Build history of the part. All positions in model axes, mm. A direction names the side the tool comes from. Give positions to 0.01 mm unless a question says otherwise; leave off trailing zeros. Write each loop counter-clockwise with the first axis right and the second up, starting at its lowest first coordinate (ties: lowest second). Pieces come first, ordered by that corner, then holes. Notation, with made-up numbers: M 15.25,7.25 L 36.25,7.25 A17 ccw 36.25,20.25 Z; hole C 0,-20.5 d4. An arc over 180 degrees is marked long. Return JSON: item names as keys, results as strings. Group by question number.
Q1. Band-saw the part on C-C, the plane y = 9.5. Give the cut face in (x, z), then the cut area to 3 significant figures.
Q2. Band-saw the part on A-A, the plane z = 0. Give the cut face in (x, y).
Q3. Tool access for faces 4 (the flat face through (-15, 6, -7.85)), 5 (the flat face through (-30, -8, 0)), 6 (the flat face through (-38.898, -8.874, 40.373)), 7 (the flat face through (-25, -15.35, 43)), 8 (the flat face through (-28.577, 15, -3)): list every direction of +Z, -Z, +X, -X, +Y, -Y with a clear straight run to the whole face (end or side of a thin tool).
Q4. Band-saw the part on B-B, the plane y = 20. Give the cut face in (x, z), then the cut area to 3 significant figures.
Q5. Band-saw the part on D-D, the plane z = 17.5. Give the cut face in (x, y), then the cut area to 3 significant figures.
Q6. Flat gauge pins, fed straight in: pin 1 Ø2 at (x, z) = (-16.5, 29) entering from +Y; pin 2 Ø7.5 at (x, y) = (-47.5, -6.5) entering from +Z; pin 3 Ø4 at (x, y) = (-40, -7.5) entering from +Z; pin 4 Ø4 at (y, z) = (2.5, 58) entering from -X. Where does each tip first touch, or does it go through?
Q7. Wall check: probe 1 along Z at (x, y) = (-4.95, 20); probe 2 along Z at (x, y) = (-44.5, -10); probe 3 along Y at (x, z) = (-60, -8.85). Give the ranges that are in metal, low to high.
Q8. Pull direction X, two halves, no side cores. Call faces 1 (the cylindrical face through (-5.43, -6.5, 0.07)), 2 (the flat face through (-42.943, -2.465, 53.109)), 3 (the cylindrical face through (-12.39, -7.3, 40.75)): +X half, -X half, draft (parallel to the pull), parting line (faces both ways), or undercut.
from build123d import *

# Parameters (mm, degrees)
F0_W      = 15
F0_H      = 15
F1_DEPTH  = 15
F2_W      = 15
F2_H      = 15
F3_DEPTH  = 3
F5_DEPTH  = 30
F6_R      = 1.5
F7_DEPTH  = 6.001
F8_R      = 1.5
F9_DEPTH  = 24.8215080757
F10_R     = 1.5
F11_DEPTH = 6.001
F12_SIZE  = 5
F13_SIZE  = 2
F14_W     = 15.7
F14_H     = 15.7
F15_DEPTH = 48.001
F16_W     = 15.7
F16_H     = 15.7
F17_DEPTH = 63.3466714755
F18_W     = 15.7
F18_H     = 15.7
F19_DEPTH = 40.001
F21_DEPTH = 18.001


with BuildPart() as f1:
    # F0 (on Front) → F1 (new body)
    with BuildSketch(Plane.XZ):
        Polygon((-70, 7.5), (-30, 7.5), (-30, -7.5), (-70, -7.5), (-70, -13.5), (-1.5766062413, -13.5), (-1.5766062413, 29.7307621135), (-23.3086570489, 67.3717782649), (-28.5048094716, 64.3717782649), (-8.5048094716, 29.7307621135), (-21.4951905284, 22.2307621135), (-41.4951905284, 56.8717782649), (-46.6913429511, 53.8717782649), (-30.8826859022, 26.4903810568), (-38.3826859022, 13.5), (-70, 13.5), align=None)
        with Locations((-15.0766062413, 0)):
            Rectangle(F0_W, F0_H, mode=Mode.SUBTRACT)
    extrude(amount=F1_DEPTH)

    # F2 (on face) → F3 (join)
    with BuildSketch(Plane.XZ.offset(15)):
        Polygon((-38.3826859022, 13.5), (-70, 13.5), (-70, -13.5), (-1.5766062413, -13.5), (-1.5766062413, 29.7307621135), (-23.3086570489, 67.3717782649), (-46.6913429511, 53.8717782649), (-30.8826859022, 26.4903810568), align=None)
        with Locations((-15.0766062413, 0)):
            Rectangle(F2_W, F2_H, mode=Mode.SUBTRACT)
    extrude(amount=F3_DEPTH)

    # F4 (on face) → F5 (join)
    with BuildSketch(Plane(origin=(0, 0, 0), x_dir=(-1, 0, 0), z_dir=(0, 1, 0))):
        Polygon((7.5766062413, -7.5), (7.5766062413, 7.5), (1.5766062413, 7.5), (1.5766062413, -13.5), (28.5766062413, -13.5), (28.5766062413, 7.5), (22.5766062413, 7.5), (22.5766062413, -7.5), align=None)
    extrude(amount=F5_DEPTH)

    # F6 (on face) → F7 (cut, through all)
    with BuildSketch(Plane.XY.offset(-7.5)):
        with Locations((-40, -7.5)):
            Circle(F6_R)
        with Locations((-60, -7.5)):
            Circle(F6_R)
    extrude(amount=-F7_DEPTH, mode=Mode.SUBTRACT)

    # F8 (on face) → F9 (cut, through all)
    with BuildSketch(Plane(origin=(6.4951905284, 0, 3.75), x_dir=(0, -1, 0), z_dir=(-0.8660254038, 0, -0.5))):
        with Locations((7.5, 40)):
            Circle(F8_R)
        with Locations((7.5, 60)):
            Circle(F8_R)
    extrude(amount=-F9_DEPTH, mode=Mode.SUBTRACT)

    # F10 (on face) → F11 (cut, through all)
    with BuildSketch(Plane(origin=(-7.5766062413, 0, 0), x_dir=(0, -1, 0), z_dir=(-1, 0, 0))):
        with Locations((-20, 0)):
            Circle(F10_R)
        with Locations((8, 0)):
            Circle(F10_R)
    extrude(amount=-F11_DEPTH, mode=Mode.SUBTRACT)

    # F12
    f12_edges = [f1.edges().sort_by_distance(p)[0] for p in [
        (-25.906733, 0, 65.871778),
        (-44.093267, 0, 55.371778),
        (-4.576606, 30, 7.5),
        (-25.576606, 30, 7.5),
        (-70, 0, 10.5),
        (-70, 0, -10.5),
    ]]
    chamfer(f12_edges, length=F12_SIZE)

    # F13
    f13_edges = [f1.edges().sort_by_distance(p)[0] for p in [
        (-1.576606, -6.5, 0),
        (-1.576606, 21.5, 0),
        (-8.308657, -6, 41.391016),
        (-18.308657, -6, 58.711524),
        (-41.5, -7.5, -13.5),
        (-61.5, -7.5, -13.5),
    ]]
    chamfer(f13_edges, length=F13_SIZE)

    # F14 (on face) → F15 (cut, through all)
    with BuildSketch(Plane.XZ.offset(18)):
        with Locations((-15.0766062413, 0)):
            Rectangle(F14_W, F14_H)
    extrude(amount=-F15_DEPTH, mode=Mode.SUBTRACT)

    # F16 (on face) → F17 (cut, through all)
    with BuildSketch(Plane(origin=(-15, 0, 25.9807621135), x_dir=(0.8660254038, 0, 0.5), z_dir=(-0.5, 0, 0.8660254038))):
        with Locations((0, -7.5)):
            Rectangle(F16_W, F16_H)
    extrude(amount=F17_DEPTH, mode=Mode.SUBTRACT)

    # F18 (on face) → F19 (cut, through all)
    with BuildSketch(Plane(origin=(-30, 0, 0), x_dir=(0, -1, 0), z_dir=(-1, 0, 0))):
        with Locations((7.5, 0)):
            Rectangle(F18_W, F18_H)
    extrude(amount=F19_DEPTH, mode=Mode.SUBTRACT)

    # F20 (on face) → F21 (cut, through all)
    with BuildSketch(Plane(origin=(0, 0, 0), x_dir=(-1, 0, 0), z_dir=(0, 1, 0))):
        Polygon((7.2266062413, 23.5405298623), (7.2266062413, 7.85), (22.9266062413, 7.85), (22.9266062413, 14.4761306361), align=None)
    extrude(amount=-F21_DEPTH, mode=Mode.SUBTRACT)


solid = f1.part
From the geometry:
{
 "1": {"outline": "M -28.58,-13.5 L -1.58,-13.5 L -1.58,7.5 L -7.23,7.5 L -7.23,-7.85 L -22.93,-7.85 L -22.93,7.5 L -28.58,7.5 Z", "area": "326 mm^2"},
 "2": {"outline": "M -70,-18 L -22.93,-18 L -22.93,30 L -28.58,30 L -28.58,0 L -30,0 L -30,-15.35 L -70,-15.35 Z; M -7.23,-18 L -1.58,-18 L -1.58,-11.5 L -3.58,-9.5 L -7.23,-9.5 Z; M -7.23,-6.5 L -3.58,-6.5 L -1.58,-4.5 L -1.58,16.5 L -3.58,18.5 L -7.23,18.5 Z; M -7.23,21.5 L -3.58,21.5 L -1.58,23.5 L -1.58,30 L -7.23,30 Z"},
 "3": {"face 4": "+Y, -Y", "face 5": "-X, +Y", "face 6": "-X, +Y, -Y", "face 7": "+Y", "face 8": "+Z, -Z, -X, +Y"},
 "4": {"outline": "M -28.58,-13.5 L -1.58,-13.5 L -1.58,-3.5 L -3.58,-1.5 L -7.23,-1.5 L -7.23,-7.85 L -22.93,-7.85 L -22.93,7.5 L -28.58,7.5 Z; M -7.23,1.5 L -3.58,1.5 L -1.58,3.5 L -1.58,7.5 L -7.23,7.5 Z", "area": "305 mm^2"},
 "5": {"outline": "M -36.07,-18 L -17.69,-18 L -17.69,0 L -36.07,0 Z; M -7.23,-18 L -1.58,-18 L -1.58,0 L -7.23,0 Z", "area": "433 mm^2"},
 "6": {"pin 1": "stops at y = -15.35", "pin 2": "stops at z = 55.57", "pin 3": "stops at z = 56.7", "pin 4": "passes through"},
 "7": {"probe 1": "z = -13.5 to -1.5, 1.5 to 7.5", "probe 2": "z = -13.5 to -7.85, 7.85 to 13.5, 50.08 to 55.14", "probe 3": "y = -18 to -9, -6 to 0"},
 "8": {"face 1": "draft", "face 2": "-X half", "face 3": "undercut"}
}
